Here's how the part is built. I have some questions about the finished solid (model axes, mm). A direction names the side the tool comes from. Round coordinates to 2 decimals unless told otherwise and drop trailing zeros. Write each loop counter-clockwise with the first axis right and the second up, starting at its lowest first coordinate (ties: lowest second). Pieces come first, ordered by that corner, then holes. Notation, with made-up numbers: (5, -37.5) -> (50, -37.5) arc R22 ccw to (50, -5.5) -> close; hole circle Ø7 at (12, -26). An arc over 180 degrees is marked (long way). Put each result on its own line as item: value. Start each with the question number.
1. I need wall thicknesses on probe 1 along Y at (x, z) = (64, 0) (3 decimals); probe 2 along Y at (x, z) = (122.5, -128.5) (3 decimals); probe 3 along X at (y, z) = (-34.5, -11). Which ranges of each line are inside material? Lowest first, please. Write a range as from..to.
2. Suppose I cut it at A-A (x = 205.5). Please give me the cut outline in (y, z) (3 decimals), then the cut area to 3 significant figures.
3. Suppose I cut it at D-D (z = -43). Please give me the cut outline in (x, y) (3 decimals).
4. For pin 1 (7.5 mm diameter, centred on y = -213, z = -80.5, fed in from -X); pin 2 (3 mm diameter, centred on x = 185.5, z = -149, fed in from -Y); pin 3 (6 mm diameter, centred on y = -29.5, z = 27, fed in from +X), each with a flat end and sliding along its axis, tell me the tip position at first contact or that it passes through.
5. Suppose I cut it at C-C (y = 0). Please give me the cut outline in (x, z) (3 decimals), then the cut area to 3 significant figures.
6. Which directions (+Z, -Z, +X, -X, +Y, -Y) give clear straight access to the entire face, cutting with the end or side of a thin tool? Please do faces 1 (the face through (249.53, -141.934, -185.756)), 2 (the face through (177, -142, 52.451)), 3 (the face through (178, -179.324, -211)), 4 (the face through (60.325, 6, -12.4)), 5 (the face through (179.578, -62.629, -143.796)).
7. Suppose I cut it at B-B (z = -117). Please give me the cut outline in (x, y) (3 decimals), then the cut area to 3 significant figures.
8. We'd pull the mould along X, two halves only. Please class faces 6 (the face through (295.275, 6, 12.4)), 7 (the face through (50.8, -202, -157)), 8 (the face through (180, -53, 52.451)): +X half, -X half, draft (parallel to the pull), parting line (faces both ways), or undercut.
```python
from build123d import *

# Parameters (mm, degrees)
SKETCH2_W           = 38.1
SKETCH2_H           = 50.8
SKETCH2_R           = 13.335
BOSS_EXTRUDE2_DEPTH = 3.175
SKETCH4_W           = 38.1
SKETCH4_H           = 50.8
SKETCH4_R           = 13.335
BOSS_EXTRUDE3_DEPTH = 3.175
BOSS_EXTRUDE4_DEPTH = 127
CUT_EXTRUDE3_DEPTH  = 127
BOSS_EXTRUDE7_DEPTH = 127
SKETCH16_R          = 38.1
BOSS_EXTRUDE8_DEPTH = 25.4
CUT_EXTRUDE6_REACH  = 522.886
SKETCH19_W          = 33.866666667
SKETCH19_H          = 115.824
SKETCH19_W_2        = 33.866666666
SKETCH20_W          = 177.8
SKETCH20_H          = 120.65
CUT_EXTRUDE7_DEPTH  = 34.925
SKETCH22_W          = 177.8
SKETCH22_H          = 118.188552156
CUT_EXTRUDE8_DEPTH  = 9.525


with BuildPart() as part:
    # Sketch2 → Boss-Extrude2 (new, symmetric)
    with BuildSketch(Plane(origin=(63.5, 0, 0), x_dir=(0, 0, -1), z_dir=(1, 0, 0))):
        Rectangle(SKETCH2_W, SKETCH2_H)
        Circle(SKETCH2_R, mode=Mode.SUBTRACT)
    extrude(amount=BOSS_EXTRUDE2_DEPTH, both=True)



with BuildPart() as body_2:
    # Sketch4 → Boss-Extrude3 (new, symmetric)
    with BuildSketch(Plane(origin=(292.1, 0, -263.652), x_dir=(0, 0, 1), z_dir=(-1, 0, 0))):
        with Locations((263.652, 0)):
            Rectangle(SKETCH4_W, SKETCH4_H)
        with Locations(Location((263.652, 0, 0), (0, 0, 180))):
            Circle(SKETCH4_R, mode=Mode.SUBTRACT)
    extrude(amount=BOSS_EXTRUDE3_DEPTH, both=True)


with BuildPart() as part_1:
    add(part.part)

    add(body_2.part)  # Boss-Extrude4 merges body 2
    # Sketch6 → Boss-Extrude4 (add, symmetric)
    with BuildSketch(Plane(origin=(177.8, 0, 0), x_dir=(0, 0, -1), z_dir=(1, 0, 0))):
        Polygon((-19.05, -25.4), (-61.976, -25.4), (-61.976, -255.524), (236.474, -255.524), (236.474, -217.424), (134.874, -25.4), (19.05, -25.4), align=None)
    extrude(amount=BOSS_EXTRUDE4_DEPTH, both=True)

    # Sketch13 → Cut-Extrude3 (cut, symmetric)
    with BuildSketch(Plane(origin=(177.8, 0, 0), x_dir=(0, 0, -1), z_dir=(1, 0, 0))):
        Polygon((-52.451, -34.925), (129.137596743, -34.925), (226.949, -219.788552156), (226.949, -255.524), (-61.976, -255.524), (-61.976, -219.788552156), (-52.451, -219.788552156), align=None)
    extrude(amount=CUT_EXTRUDE3_DEPTH, both=True, mode=Mode.SUBTRACT)

    # Sketch14 → Boss-Extrude7 (add, symmetric)
    with BuildSketch(Plane(origin=(177.8, 0, 0), x_dir=(0, 0, -1), z_dir=(1, 0, 0))):
        Polygon((226.949, -219.788552156), (-52.451, -219.788552156), (-52.451, -210.263552156), (221.90931746, -210.263552156), align=None)
        Polygon((-52.451, -146.763552156), (188.311433862, -146.763552156), (183.271751323, -137.238552156), (-52.451, -137.238552156), align=None)
    extrude(amount=BOSS_EXTRUDE7_DEPTH, both=True)

    # Sketch16 → Boss-Extrude8 (add)
    with BuildSketch(Plane(origin=(304.8, 0, 0), x_dir=(0, 0, -1), z_dir=(1, 0, 0))):
        with Locations(Location((-23.876, -232.488552156, 0), (0, 0, 160.528779366))):
            Circle(SKETCH16_R)
        with Locations(Location((160.274, -232.488552156, 0), (0, 0, 160.528779366))):
            Circle(SKETCH16_R)
    boss_extrude8 = extrude(amount=BOSS_EXTRUDE8_DEPTH)

    # Mirror1: Boss-Extrude8 across plane
    add(boss_extrude8.mirror(Plane(origin=(177.8, 0, 0), x_dir=(0, 0, 1), z_dir=(1, 0, 0))))

    # Cut-Extrude6: up to this plane
    cut_extrude6_end = Plane(origin=(50.8, -34.925, -129.137596743), z_dir=(0, 0.46767282988430103, -0.8839016484813284))
    # Sketch19 → Cut-Extrude6 (cut, up to the surface)
    with BuildSketch(Plane(origin=(0, 0, -236.474), x_dir=(-1, 0, 0), z_dir=(0, 0, -1)), mode=Mode.PRIVATE) as cut_extrude6_sk1:
        with Locations((-249.766666666, -121.412)):
            Rectangle(SKETCH19_W, SKETCH19_H)
    cut_extrude6_tool1 = split(extrude(cut_extrude6_sk1.sketch, amount=-CUT_EXTRUDE6_REACH, mode=Mode.PRIVATE), bisect_by=cut_extrude6_end, keep=Keep.BOTH, mode=Mode.PRIVATE)
    add(cut_extrude6_tool1.solids().sort_by_distance((249.766667, -121.412, -236.474))[0], mode=Mode.SUBTRACT)
    # Sketch19 → Cut-Extrude6 (cut, up to the surface)
    with BuildSketch(Plane(origin=(0, 0, -236.474), x_dir=(-1, 0, 0), z_dir=(0, 0, -1)), mode=Mode.PRIVATE) as cut_extrude6_sk2:
        with Locations((-177.8, -121.412)):
            Rectangle(SKETCH19_W_2, SKETCH19_H)
    cut_extrude6_tool2 = split(extrude(cut_extrude6_sk2.sketch, amount=-CUT_EXTRUDE6_REACH, mode=Mode.PRIVATE), bisect_by=cut_extrude6_end, keep=Keep.BOTH, mode=Mode.PRIVATE)
    add(cut_extrude6_tool2.solids().sort_by_distance((177.8, -121.412, -236.474))[0], mode=Mode.SUBTRACT)
    # Sketch19 → Cut-Extrude6 (cut, up to the surface)
    with BuildSketch(Plane(origin=(0, 0, -236.474), x_dir=(-1, 0, 0), z_dir=(0, 0, -1)), mode=Mode.PRIVATE) as cut_extrude6_sk3:
        with Locations((-105.833333334, -121.412)):
            Rectangle(SKETCH19_W, SKETCH19_H)
    cut_extrude6_tool3 = split(extrude(cut_extrude6_sk3.sketch, amount=-CUT_EXTRUDE6_REACH, mode=Mode.PRIVATE), bisect_by=cut_extrude6_end, keep=Keep.BOTH, mode=Mode.PRIVATE)
    add(cut_extrude6_tool3.solids().sort_by_distance((105.833333, -121.412, -236.474))[0], mode=Mode.SUBTRACT)

    # Sketch20 → Cut-Extrude7 (cut)
    with BuildSketch(Plane(origin=(0, 0, 0), x_dir=(1, 0, 0), z_dir=(0, 1, 0))):
        with Locations((177.8, 36.449)):
            Rectangle(SKETCH20_W, SKETCH20_H)
    extrude(amount=-CUT_EXTRUDE7_DEPTH, mode=Mode.SUBTRACT)

    # Sketch22 → Cut-Extrude8 (cut)
    with BuildSketch(Plane.XY.offset(61.976)):
        with Locations((177.8, -122.594276078)):
            Rectangle(SKETCH22_W, SKETCH22_H)
    extrude(amount=-CUT_EXTRUDE8_DEPTH, mode=Mode.SUBTRACT)


solid = part_1.part
```
Verdict:
1. probe 1: y = -219.789..-210.264, -146.764..-137.239, -34.925..-13.335, 13.335..25.4
1. probe 2: y = -219.789..-210.264, -146.764..-137.239, -34.925..-25.4
1. probe 3: x = 50.8..88.9, 266.7..304.8
2. outline: (-255.524, -236.474) -> (-217.424, -236.474) -> (-25.4, -134.874) -> (-25.4, -96.774) -> (-34.925, -96.774) -> (-34.925, -129.138) -> (-137.239, -183.272) -> (-137.239, 52.451) -> (-146.764, 52.451) -> (-146.764, -188.311) -> (-210.264, -221.909) -> (-210.264, 52.451) -> (-181.689, 52.451) -> (-181.689, 61.976) -> (-219.789, 61.976) -> (-219.789, -226.949) -> (-255.524, -226.949) -> close; (-63.5, 52.451) -> (-34.925, 52.451) -> (-34.925, 23.876) -> (-25.4, 23.876) -> (-25.4, 61.976) -> (-63.5, 61.976) -> close
2. area: 8,620 mm^2
3. outline: (50.8, -219.789) -> (304.8, -219.789) -> (304.8, -210.264) -> (50.8, -210.264) -> close; (50.8, -146.764) -> (304.8, -146.764) -> (304.8, -137.239) -> (50.8, -137.239) -> close; (50.8, -34.925) -> (88.9, -34.925) -> (88.9, -25.4) -> (50.8, -25.4) -> close; (266.7, -34.925) -> (304.8, -34.925) -> (304.8, -25.4) -> (266.7, -25.4) -> close
4. pin 1: stops at x = 50.8
4. pin 2: stops at y = -219.79
4. pin 3: stops at x = 304.8
5. outline: (60.325, -19.05) -> (66.675, -19.05) -> (66.675, -13.335) -> (60.325, -13.335) -> close; (60.325, 13.335) -> (66.675, 13.335) -> (66.675, 19.05) -> (60.325, 19.05) -> close; (288.925, -19.05) -> (295.275, -19.05) -> (295.275, -13.335) -> (288.925, -13.335) -> close; (288.925, 13.335) -> (295.275, 13.335) -> (295.275, 19.05) -> (288.925, 19.05) -> close
5. area: 145 mm^2
6. face 1: -Z, +Y
6. face 2: +Z
6. face 3: +Z, -Z, +Y
6. face 4: +Z, -Z, -X, +Y
6. face 5: +X, -X
7. outline: (50.8, -219.789) -> (304.8, -219.789) -> (304.8, -210.264) -> (50.8, -210.264) -> close; (50.8, -146.764) -> (304.8, -146.764) -> (304.8, -137.239) -> (50.8, -137.239) -> close; (50.8, -34.925) -> (304.8, -34.925) -> (304.8, -25.4) -> (50.8, -25.4) -> close
7. area: 7,260 mm^2
8. face 6: +X half
8. face 7: undercut
8. face 8: draft
